The model under review builds one solid part; all positions refer to its coordinate system, in mm. A direction names the side the tool comes from. Coordinates: 2 decimals unless noted, no trailing zeros. Order: outer loops, then holes, each group sorted by start corner. A loop starts at its lowest first (then second) coordinate and runs counter-clockwise, first axis right, second up. Notation, with made-up numbers: M 14,-6 L 21,-6 A23 ccw 21,6 Z; hole C 46,79.5 d2. An arc over 180 degrees is marked long. Answer as CSV lines item,"result". Start each with the question number.
Q1. Consider section A-A on y = 0. Write out the cut boundary in (x, z), and give its area (3 significant figures).
Q2. The part is to be moulded in two halves that separate along Y. For faces 1 (the face through (43.545, 68.3, 1.479)), 2 (the face through (-1, -53, 3)), 3 (the face through (42.397, 13.352, 14.399)), say which applies: +Y half, -Y half, draft (parallel to the pull), parting line (faces both ways), or undercut.
Q3. Consider section C-C on z = 21.5. Write out the cut boundary in (x, y), and give its area (3 significant figures).
Q4. For P1, Ø4, axis at x = 46, z = 18.5, coming from the -Y side; P2, Ø2, axis at y = 8, z = 12.5, coming from the -X side; P3, Ø3, axis at x = -37.5, z = 23, coming from the -Y side, all flat-tipped, find the tip position at first contact; note any pin that passes through.
Q5. Consider section D-D on x = 55.5. Write out the cut boundary in (y, z).
Q6. Machinability: for faces 4 (the face through (35, -35, 0)), 5 (the face through (-11.012, -49.592, 15.522)), which of the approach directions +Z, -Z, +X, -X, +Y, -Y give a long, thin tool a straight path to every point of the face, cutting with its end or side? Answer none if there is none.
Q7. Wall thickness on L1, parallel to Y at x = 0, z = 18; L2, parallel to X at y = -26, z = 8; L3, parallel to Z at x = 32.5, y = -61: over which ranges is each line inside the solid? List them lowest first. Write a range as [from, to].
from build123d import *

# Parameters (mm, degrees)
F0_R     = 81
F1_DEPTH = 3
F2_R     = 50.8
F3_DEPTH = 25.4
F4_R     = 44.45
F5_DEPTH = 28.401


with BuildPart() as f1:
    # F0 (on Top) → F1 (new body)
    with BuildSketch(Plane.XY):
        Circle(F0_R)
    extrude(amount=F1_DEPTH)

    # F2 (on face) → F3 (join)
    with BuildSketch(Plane.XY.offset(3)):
        Circle(F2_R)
    extrude(amount=F3_DEPTH)

    # F4 (on face) → F5 (cut, through all)
    with BuildSketch(Plane.XY.offset(28.4)):
        Circle(F4_R)
    extrude(amount=-F5_DEPTH, mode=Mode.SUBTRACT)


solid = f1.part
Evaluation:
1,outline,"M -81,0 L -44.45,0 L -44.45,28.4 L -50.8,28.4 L -50.8,3 L -81,3 Z; M 44.45,0 L 81,0 L 81,3 L 50.8,3 L 50.8,28.4 L 44.45,28.4 Z"
1,area,"542 mm²"
2,face 1,"parting line"
2,face 2,"draft"
2,face 3,"undercut"
3,outline,"C 0,0 d101.6; hole C 0,0 d88.9"
3,area,"1,900 mm²"
4,P1,"stops at y = -25.39"
4,P2,"stops at x = -50.32"
4,P3,"stops at y = -35.84"
5,outline,"M -59,0 L 59,0 L 59,3 L -59,3 Z"
6,face 4,"-Z, +X, -X, +Y, -Y"
6,face 5,"+Z"
7,L1,"y = [-50.8, -44.45], [44.45, 50.8]"
7,L2,"x = [-43.64, -36.05], [36.05, 43.64]"
7,L3,"z = [0, 3]"
